Input: part model. Units: mm. Frame: model coordinates. Face numbers are marked on the shaded views. A direction names the side the tool comes from. Round coordinates to 2 decimals unless told otherwise and drop trailing zeros. Order: outer loops, then holes, each group sorted by start corner. A loop starts at its lowest first (then second) coordinate and runs counter-clockwise, first axis right, second up. Notation, with made-up numbers: (-7.75, -16.5) -> (7.25, -16.5) arc R25 cw to (7.25, 12.5) -> close; hole circle Ø8 at (27, 10.5). An arc over 180 degrees is marked (long way). Use a Markdown table: item, result.
from build123d import *

# Parameters (mm, degrees)
SKETCH1_W           = 100
SKETCH1_H           = 15
BODY_DEPTH          = 15
CLICK_DEPTH         = 7
CLICK_CHAMFER_SIZE  = 1
SKETCH3_W           = 92
SKETCH3_H           = 13
CUT_EXTRUDE1_DEPTH  = 13
SKETCH4_R           = 3.5
CUT_EXTRUDE2_DEPTH  = 13
SKETCH5_W           = 10.75
SKETCH5_H           = 12
CUT_EXTRUDE3_DEPTH  = 10
SKETCH6_W           = 10.75
SKETCH6_H           = 13
BOSS_EXTRUDE1_DEPTH = 1
SKETCH7_W           = 2
SKETCH7_H           = 13
BOSS_EXTRUDE2_DEPTH = 13
SKETCH8_W           = 2
SKETCH8_H           = 5
BOSS_EXTRUDE3_DEPTH = 13


with BuildPart() as part:
    # Sketch1 → Body (new body)
    with BuildSketch(Plane.XY):
        Rectangle(SKETCH1_W, SKETCH1_H)
    extrude(amount=BODY_DEPTH)

    # Sketch2 → Click (add)
    with BuildSketch(Plane.XY):
        Polygon((-50, 0), (-50, 2.45), (-57.45, 4.95), (-57.45, 0), (-57.45, -4.95), (-50, -2.45), align=None)
        Polygon((57.45, 0), (57.45, -4.95), (50, -2.45), (50, 0), (50, 2.45), (57.45, 4.95), align=None)
    extrude(amount=CLICK_DEPTH)

    # Click Chamfer
    click_chamfer_edges = [part.edges().sort_by_distance(p)[0] for p in [
        (-50, 0, 15),
        (50, 0, 15),
    ]]
    chamfer(click_chamfer_edges, length=CLICK_CHAMFER_SIZE)

    # Sketch3 → Cut-Extrude1 (cut)
    with BuildSketch(Plane.XZ.offset(7.5)):
        with Locations((0, 6.5)):
            Rectangle(SKETCH3_W, SKETCH3_H)
    extrude(amount=-CUT_EXTRUDE1_DEPTH, mode=Mode.SUBTRACT)

    # Sketch4 → Cut-Extrude2 (cut)
    with BuildSketch(Plane.XY.offset(15)):
        with Locations((-16.8, 0)):
            Circle(SKETCH4_R)
        with Locations((-36.4, 0)):
            Circle(SKETCH4_R)
        with Locations((16.8, 0)):
            Circle(SKETCH4_R)
        with Locations((36.4, 0)):
            Circle(SKETCH4_R)
    extrude(amount=-CUT_EXTRUDE2_DEPTH, mode=Mode.SUBTRACT)

    # Sketch5 → Cut-Extrude3 (cut)
    with BuildSketch(Plane(origin=(0, 7.5, 0), x_dir=(1, 0, 0), z_dir=(0, 1, 0))):
        with Locations((0, -6)):
            Rectangle(SKETCH5_W, SKETCH5_H)
    extrude(amount=-CUT_EXTRUDE3_DEPTH, mode=Mode.SUBTRACT)

    # Sketch6 → Boss-Extrude1 (add)
    with BuildSketch(Plane(origin=(0, 0, 13), x_dir=(-1, 0, 0), z_dir=(0, 0, -1))):
        with Locations((0, -1)):
            Rectangle(SKETCH6_W, SKETCH6_H)
    extrude(amount=BOSS_EXTRUDE1_DEPTH)

    # Sketch7 → Boss-Extrude2 (add)
    with BuildSketch(Plane(origin=(0, 0, 13), x_dir=(-1, 0, 0), z_dir=(0, 0, -1))):
        with Locations((6.375, -1)):
            Rectangle(SKETCH7_W, SKETCH7_H)
    extrude(amount=BOSS_EXTRUDE2_DEPTH)

    # Sketch8 → Boss-Extrude3 (add)
    with BuildSketch(Plane(origin=(0, 0, 13), x_dir=(-1, 0, 0), z_dir=(0, 0, -1))):
        with Locations((-6.375, 3)):
            Rectangle(SKETCH8_W, SKETCH8_H)
    extrude(amount=BOSS_EXTRUDE3_DEPTH)


solid = part.part
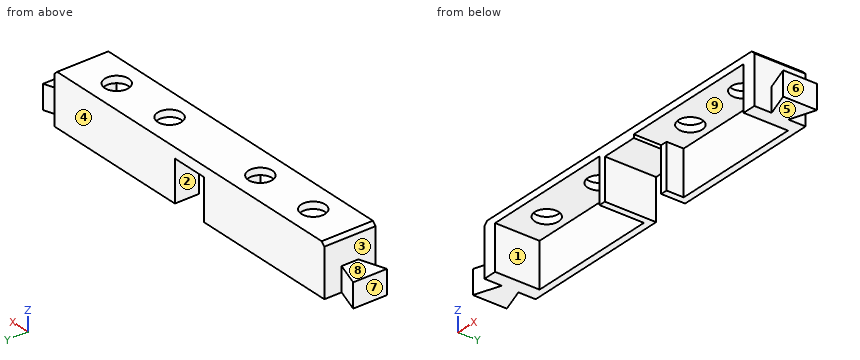
1) Cut plane A-A on z = 4. Return loops of the section in (x, y) (3 decimals), and give its area (3 significant figures).
Results found:
| item | result |
|---|---|
| outline | (-57.45, -4.95) -> (-50, -2.45) -> (-50, -7.5) -> (-46, -7.5) -> (-46, 5.5) -> (-7.375, 5.5) -> (-7.375, -7.5) -> (-5.375, -7.5) -> (-5.375, 7.5) -> (-50, 7.5) -> (-50, 2.45) -> (-57.45, 4.95) -> close; (5.375, 0.5) -> (7.375, 0.5) -> (7.375, 5.5) -> (46, 5.5) -> (46, -7.5) -> (50, -7.5) -> (50, -2.45) -> (57.45, -4.95) -> (57.45, 4.95) -> (50, 2.45) -> (50, 7.5) -> (5.375, 7.5) -> close |
| area | 429 mm² |
2) Cut plane C-C on y = -6. Return loops of the section in (x, z) (3 decimals).
Results found:
| item | result |
|---|---|
| outline | (-50, 0) -> (-46, 0) -> (-46, 13) -> (-7.375, 13) -> (-7.375, 0) -> (-5.375, 0) -> (-5.375, 12) -> (5.375, 12) -> (5.375, 13) -> (46, 13) -> (46, 0) -> (50, 0) -> (50, 14) -> (49, 15) -> (-49, 15) -> (-50, 14) -> close |
3) Pull-direction query (X, two-part tool) for the marked faces 6, 7, 8 and 9; classes: +X half, -X half, draft (parallel to the pull), parting line (faces both ways), or undercut.
Results found:
| item | result |
|---|---|
| face 6 | +X half |
| face 7 | -X half |
| face 8 | draft |
| face 9 | undercut |
4) Set-up query: the marked faces 1, 2, 3, 4 and 5. Return all of +Z, -Z, +X, -X, +Y, -Y with unobstructed straight access to the full face (end or side cutting, diameter ignored); none if empty.
Results found:
| item | result |
|---|---|
| face 1 | -Z, -Y |
| face 2 | -Z, +Y, -Y |
| face 3 | +Z |
| face 4 | +Z, -Z, +X, -X, +Y |
| face 5 | -Z, +X, -X, +Y, -Y |
5) Cut plane B-B on x = 16.8. Return loops of the section in (y, z), and give its area (3 significant figures).
Results found:
| item | result |
|---|---|
| outline | (-7.5, 13) -> (-3.5, 13) -> (-3.5, 15) -> (-7.5, 15) -> close; (3.5, 13) -> (5.5, 13) -> (5.5, 0) -> (7.5, 0) -> (7.5, 15) -> (3.5, 15) -> close |
| area | 42.0 mm² |
6) Line query: L1, parallel to X at y = -6.25, z = 4 (3 decimals); L2, parallel to X at y = 1.5, z = 8 (3 decimals); L3, parallel to Y at x = -36.4, z = 13.7. Output: solid intervals per line, ascending. Write a range as [from, to].
Results found:
| item | result |
|---|---|
| L1 | x = [-50, -46], [-7.375, -5.375], [46, 50] |
| L2 | x = [-50, -46], [-7.375, -5.375], [5.375, 7.375], [46, 50] |
| L3 | y = [-7.5, -3.5], [3.5, 7.5] |
7) Cut plane D-D on z = 10.5. Return loops of the section in (x, y) (3 decimals), and give its area (4 significant figures).
Results found:
| item | result |
|---|---|
| outline | (-50, -7.5) -> (-46, -7.5) -> (-46, 5.5) -> (-7.375, 5.5) -> (-7.375, -7.5) -> (-5.375, -7.5) -> (-5.375, 7.5) -> (-50, 7.5) -> close; (5.375, 0.5) -> (7.375, 0.5) -> (7.375, 5.5) -> (46, 5.5) -> (46, -7.5) -> (50, -7.5) -> (50, 7.5) -> (5.375, 7.5) -> close |
| area | 318.5 mm² |
8) Pin query (flat end, axial travel): pin 1 Ø1 at (x, z) = (-29.5, 7.5) entering from -Y; pin 2 Ø1.1 at (y, z) = (-2.5, 12.5) entering from +X; pin 3 Ø2 at (x, y) = (54, -1) entering from +Z. Return the tip coordinate at first contact, or that it passes through.
Results found:
| item | result |
|---|---|
| pin 1 | stops at y = 5.5 |
| pin 2 | stops at x = 50 |
| pin 3 | stops at z = 7 |
